Autodesk Inventor part; units mm, degrees
ref_plane "YZ Plane" through (0, 0, 0) normal (1, 0, 0) x (0, 1, 0)
ref_plane "XZ Plane" through (0, 0, 0) normal (0, 1, 0) x (-1, 0, 0)
ref_plane "XY Plane" through (0, 0, 0) normal (0, 0, 1) x (1, 0, 0)
sketch "Sketch1" plane through (0, 0, 0) normal (1, 0, 0) x (0, 1, 0)
  line L0 (0, 0) -> (7, 0) construction
  line L1 (7, 0) -> (7, -17.5) construction
  line L2 (7, -17.5) -> (0, -17.5)
  line L3 (0, -17.5) -> (0, 0) construction
  line L4 (7, -23.5) -> (0, -23.5)
  line L5 (7, -18.5) -> (6.8, -18.5)
  line L6 (6.8, -18.5) -> (6.8, -22.5)
  line L7 (6.8, -22.5) -> (7, -22.5)
  line L8 (0, -18.5) -> (0.2, -18.5)
  line L9 (0.2, -18.5) -> (0.2, -22.5)
  line L10 (0.2, -22.5) -> (0, -22.5)
  line L11 (7, -17.5) -> (7, -18.5)
  line L12 (7, -22.5) -> (7, -23.5)
  line L13 (0, -23.5) -> (0, -22.5)
  line L14 (0, -18.5) -> (0, -17.5)
  dimension "d0" = 17.5
  dimension "d2" = 7
  dimension "d5" = 23.5
  dimension "d6" = 0.2
  dimension "d7" = 1
revolve "Revolution1" add sketch "Sketch1" angle 360 about axis through (0, 0, 0) along (0, 1, 0)
properties part number "6807 bearing"
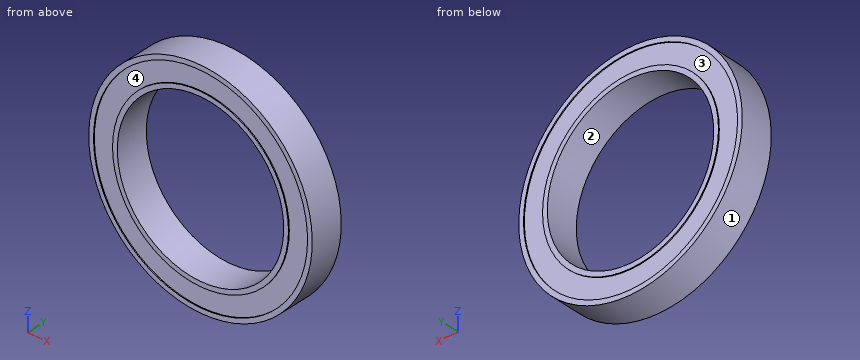
CAD build for the part. Positions are in the model's coordinates, mm. Face numbers are marked on the shaded views. A direction names the side the tool comes from. Give positions to 0.01 mm unless a question says otherwise; leave off trailing zeros. Write each loop counter-clockwise with the first axis right and the second up, starting at its lowest first coordinate (ties: lowest second). Pieces come first, ordered by that corner, then holes. Notation, with made-up numbers: M 25.25,41.25 L 61.25,41.25 A10 cw 61.25,48.25 Z; hole C -24.75,18 d6. An arc over 180 degrees is marked long. Put each result on its own line as item: value. Start each with the question number.
(1) Which spindle directions (+Z, -Z, +X, -X, +Y, -Y) get a long thin tool onto all of the face, cutting with end or side? Do the marked faces 3 and 4. Say none if no direction does.
(2) Probe L1, parallel to X at y = 6.95, z = 0; L2, parallel to X at y = 3.25, z = -0.5. List the from-to ranges inside material, lowest first.
(3) Band-saw the part on B-B, the plane x = 0. Write the cut outline in (y, z), and give its area (3 significant figures).
(4) Band-saw the part on A-A, the plane z = 0. Write the cut outline in (x, y), and give its area (3 significant figures).
(5) Band-saw the part on C-C, the plane y = 1.5. Write the cut outline in (x, z).
(6) Mould opens along X. For the marked faces 1 and 2 say: +X half, -X half, draft (parallel to the pull), parting line (faces both ways), or undercut.
(7) Flat gauge pins, fed straight in: pin 1 Ø1.5 at (x, y) = (16.5, 3.5) entering from +Z; pin 2 Ø1.5 at (x, y) = (-10, 6) entering from -Z; pin 3 Ø1 at (y, z) = (5, 7.5) entering from +X. Where does each tip first touch, or does it go through?
Response values:
1. face 3: +Y
1. face 4: -Y
2. L1: x = -23.5 to -22.5, -18.5 to -17.5, 17.5 to 18.5, 22.5 to 23.5
2. L2: x = -23.49 to -17.49, 17.49 to 23.49
3. outline: M 0,-23.5 L 7,-23.5 L 7,-22.5 L 6.8,-22.5 L 6.8,-18.5 L 7,-18.5 L 7,-17.5 L 0,-17.5 L 0,-18.5 L 0.2,-18.5 L 0.2,-22.5 L 0,-22.5 Z; M 0,17.5 L 7,17.5 L 7,18.5 L 6.8,18.5 L 6.8,22.5 L 7,22.5 L 7,23.5 L 0,23.5 L 0,22.5 L 0.2,22.5 L 0.2,18.5 L 0,18.5 Z
3. area: 80.8 mm2
4. outline: M -23.5,0 L -22.5,0 L -22.5,0.2 L -18.5,0.2 L -18.5,0 L -17.5,0 L -17.5,7 L -18.5,7 L -18.5,6.8 L -22.5,6.8 L -22.5,7 L -23.5,7 Z; M 17.5,0 L 18.5,0 L 18.5,0.2 L 22.5,0.2 L 22.5,0 L 23.5,0 L 23.5,7 L 22.5,7 L 22.5,6.8 L 18.5,6.8 L 18.5,7 L 17.5,7 Z
4. area: 80.8 mm2
5. outline: C 0,0 d47; hole C 0,0 d35
6. face 1: parting line
6. face 2: undercut
7. pin 1: stops at z = 17.44
7. pin 2: stops at z = -21.6
7. pin 3: stops at x = 22.43
